from build123d import *

# Parameters (mm, degrees)
ESBO_O1_W                = 150
ESBO_O1_H                = 150
ESBO_O1_R                = 2.5
RESSALTO_EXTRUS_O1_DEPTH = 6
CORTE_EXTRUS_O1_DEPTH    = 6
ESBO_O3_W                = 70
ESBO_O3_H                = 50
CORTE_EXTRUS_O2_DEPTH    = 6
FILETE1_R                = 5
ESBO_O4_R                = 1.5
CORTE_EXTRUS_O3_DEPTH    = 6


with BuildPart() as part:
    # Esboço1 → Ressalto-extrusão1 (new body)
    with BuildSketch(Plane.XY):
        with Locations((-63.750118326, 45.053956835)):
            Rectangle(ESBO_O1_W, ESBO_O1_H)
        with Locations((-83.750118326, 65.053956835)):
            Circle(ESBO_O1_R, mode=Mode.SUBTRACT)
        with Locations((-83.750118326, 25.053956835)):
            Circle(ESBO_O1_R, mode=Mode.SUBTRACT)
        with Locations((-43.750118326, 45.053956835)):
            Circle(ESBO_O1_R, mode=Mode.SUBTRACT)
    extrude(amount=RESSALTO_EXTRUS_O1_DEPTH)

    # Esboço2 → Corte-extrusão1 (cut)
    with BuildSketch(Plane.XY.offset(6)):
        Polygon((-8.750118326, 120.053956835), (-20.29712371, 100.053956835), (-107.203112943, 100.053956835), (-118.750118326, 120.053956835), align=None)
    extrude(amount=-CORTE_EXTRUS_O1_DEPTH, mode=Mode.SUBTRACT)

    # Esboço3 → Corte-extrusão2 (cut)
    with BuildSketch(Plane.XY.offset(6)):
        with Locations((-23.750118326, -4.946043165)):
            Rectangle(ESBO_O3_W, ESBO_O3_H)
    extrude(amount=-CORTE_EXTRUS_O2_DEPTH, mode=Mode.SUBTRACT)

    # Filete1
    filete1_edges = [part.edges().sort_by_distance(p)[0] for p in [
        (-20.29712371, 100.053956835, 3),
        (-107.203112943, 100.053956835, 3),
        (-118.750118326, 120.053956835, 3),
        (-8.750118326, 120.053956835, 3),
        (-58.750118326, -29.946043165, 3),
        (-58.750118326, 20.053956835, 3),
        (11.249881674, 20.053956835, 3),
        (-138.750118326, -29.946043165, 3),
        (-138.750118326, 120.053956835, 3),
        (11.249881674, 120.053956835, 3),
    ]]
    fillet(filete1_edges, radius=FILETE1_R)

    # Esboço4 → Corte-extrusão3 (cut)
    with BuildSketch(Plane.XY.offset(6)):
        with Locations((1.249881674, 110.053956835)):
            Circle(ESBO_O4_R)
        with Locations((1.249881674, 30.053956835)):
            Circle(ESBO_O4_R)
        with Locations((-128.750118326, 110.053956835)):
            Circle(ESBO_O4_R)
        with Locations((-128.750118326, -19.946043165)):
            Circle(ESBO_O4_R)
    extrude(amount=-CORTE_EXTRUS_O3_DEPTH, mode=Mode.SUBTRACT)


solid = part.part
For this review, take the finished solid that the model builds, in its own axes (mm). A direction names the side the tool comes from. Round coordinates to 2 decimals unless told otherwise and drop trailing zeros. Loops run counter-clockwise (first coordinate to the right, second up) from the corner with the lowest first, then second, coordinate; pieces in that order, holes last. Notation, with made-up numbers: (-36, 53) - (-6, 53) arc R34 cw to (-6, 89) - close; hole circle Ø3 at (0, 45). An arc over 180 degrees is marked (long way). Put each result on its own line as item: value. Start each with the question number.
1. Consider section A-A on z = 4.5. State the section outline as (x, y) points.
2. Mouldability with a two-part tool opening along X and no side actions: class faces 1 (the flat face through (-128, 120.054, 3)), 2 (the cylindrical face through (-106.848, 100.742, 2.958)), 3 (the cylindrical face through (-137.324, -28.442, 3.042)) as +X half, -X half, draft (parallel to the pull), parting line (faces both ways), or undercut.
3. For faces 4 (the cylindrical face through (-20.716, 100.706, 2.958)), 5 (the cylindrical face through (-86.248, 65.164, 2.958)), 6 (the flat face through (-58.75, -5, 3)), list the 3-axis set-ups (+Z, -Z, +X, -X, +Y, -Y) from which the entire face can be reached by the end or side of a thin tool; tool diameter is ignored.
4. Consider section D-D on x = -51.5. State the section outline as (y, z) points.
5. For probe 1 along Y at (x, z) = (-84, 0.65); probe 2 along X at (y, z) = (105, 2.4); probe 3 along Y at (x, z) = (-29, 4.5), list the stretches that pass through material, from the lowest coordinate up. Write a range as [from, to].
6. Insertion check: P1, Ø1.8, axis at y = -2, z = 3, coming from the +X side; P2, Ø6, axis at x = -8, y = 33, coming from the -Z side; P3, Ø1.8, axis at x = -29.5, z = 2.5, coming from the -Y side. Each pin has a flat end and moves straight along its axis. Give the tip position at first contact, or say it passes through.
7. Consider section C-C on y = 10. State the section outline as (x, z) points, plus the area to 3 significant figures.
8. Consider section B-B on x = -84. State the section outline as (y, z) points.
Result sheet:
1. outline: (-138.75, -24.95) arc R5 ccw to (-133.75, -29.95) - (-63.75, -29.95) arc R5 ccw to (-58.75, -24.95) - (-58.75, 15.05) arc R5 cw to (-53.75, 20.05) - (6.25, 20.05) arc R5 ccw to (11.25, 25.05) - (11.25, 115.05) arc R5 ccw to (6.25, 120.05) - (-5.86, 120.05) arc R5 ccw to (-10.19, 117.55) - (-18.85, 102.55) arc R5 cw to (-23.18, 100.05) - (-104.32, 100.05) arc R5 cw to (-108.65, 102.55) - (-117.31, 117.55) arc R5 ccw to (-121.64, 120.05) - (-133.75, 120.05) arc R5 ccw to (-138.75, 115.05) - close; hole circle Ø3 at (-128.75, -19.95); hole circle Ø3 at (-128.75, 110.05); hole circle Ø5 at (-83.75, 25.05); hole circle Ø5 at (-83.75, 65.05); hole circle Ø5 at (-43.75, 45.05); hole circle Ø3 at (1.25, 30.05); hole circle Ø3 at (1.25, 110.05)
2. face 1: draft
2. face 2: undercut
2. face 3: -X half
3. face 4: +Z, -Z, +Y
3. face 5: +Z, -Z
3. face 6: +Z, -Z, +X, -Y
4. outline: (20.05, 0) - (100.05, 0) - (100.05, 6) - (20.05, 6) - close
5. probe 1: [-29.95, 22.57], [27.54, 62.57], [67.54, 100.05]
5. probe 2: [-138.75, -110.06], [-17.44, 11.25]
5. probe 3: [20.05, 100.05]
6. P1: x = -58.75
6. P2: z = 0
6. P3: y = 20.05
7. outline: (-138.75, 0) - (-58.75, 0) - (-58.75, 6) - (-138.75, 6) - close
7. area: 480 mm^2
8. outline: (-29.95, 0) - (22.57, 0) - (22.57, 6) - (-29.95, 6) - close; (27.54, 0) - (62.57, 0) - (62.57, 6) - (27.54, 6) - close; (67.54, 0) - (100.05, 0) - (100.05, 6) - (67.54, 6) - close
